Part model, mm, in its own coordinate system. Give positions to 0.01 mm unless a question says otherwise; leave off trailing zeros. One line per question, with ' | ' between items.
```python
from build123d import *

# Parameters (mm, degrees)
SKETCH1_R           = 2.5
BOSS_EXTRUDE1_DEPTH = 240


with BuildPart() as part:
    # Sketch1 → Boss-Extrude1 (new, symmetric)
    with BuildSketch(Plane(origin=(0, 0, 0), x_dir=(1, 0, 0), z_dir=(0, 1, 0))):
        with BuildLine():
            Line((-2.185786438, 3.6), (2.185786438, 3.6))
            Line((2.185786438, 3.6), (5.5, 6.914213562))
            Line((5.5, 6.914213562), (5.5, 8))
            Line((5.5, 8), (3, 8))
            Line((3, 8), (3, 10))
            Line((3, 10), (17, 10))
            Line((17, 10), (17, 8))
            Line((17, 8), (14.5, 8))
            Line((14.5, 8), (14.5, 6.914213562))
            Line((14.5, 6.914213562), (17.814213562, 3.6))
            Line((17.814213562, 3.6), (22.185786438, 3.6))
            Line((22.185786438, 3.6), (25.5, 6.914213562))
            Line((25.5, 6.914213562), (25.5, 8))
            Line((25.5, 8), (23, 8))
            Line((23, 8), (23, 10))
            Line((23, 10), (28.5, 10))
            ThreePointArc((28.5, 10), (29.560660172, 9.560660172), (30, 8.5))
            Line((30, 8.5), (30, 3))
            Line((30, 3), (28, 3))
            Line((28, 3), (28, 5.5))
            Line((28, 5.5), (26.914213562, 5.5))
            Line((26.914213562, 5.5), (23.914213562, 2.5))
            Line((23.914213562, 2.5), (23.914213562, -2.5))
            Line((23.914213562, -2.5), (26.914213562, -5.5))
            Line((26.914213562, -5.5), (28, -5.5))
            Line((28, -5.5), (28, -3))
            Line((28, -3), (30, -3))
            Line((30, -3), (30, -8.5))
            ThreePointArc((30, -8.5), (29.560660172, -9.560660172), (28.5, -10))
            Line((28.5, -10), (23, -10))
            Line((23, -10), (23, -8))
            Line((23, -8), (25.5, -8))
            Line((25.5, -8), (25.5, -6.914213562))
            Line((25.5, -6.914213562), (22.185786438, -3.6))
            Line((22.185786438, -3.6), (17.814213562, -3.6))
            Line((17.814213562, -3.6), (14.5, -6.914213562))
            Line((14.5, -6.914213562), (14.5, -8))
            Line((14.5, -8), (17, -8))
            Line((17, -8), (17, -10))
            Line((17, -10), (3, -10))
            Line((3, -10), (3, -8))
            Line((3, -8), (5.5, -8))
            Line((5.5, -8), (5.5, -6.914213562))
            Line((5.5, -6.914213562), (2.185786438, -3.6))
            Line((2.185786438, -3.6), (-2.185786438, -3.6))
            Line((-2.185786438, -3.6), (-5.5, -6.914213562))
            Line((-5.5, -6.914213562), (-5.5, -8))
            Line((-5.5, -8), (-3, -8))
            Line((-3, -8), (-3, -10))
            Line((-3, -10), (-17, -10))
            Line((-17, -10), (-17, -8))
            Line((-17, -8), (-14.5, -8))
            Line((-14.5, -8), (-14.5, -6.914213562))
            Line((-14.5, -6.914213562), (-17.814213562, -3.6))
            Line((-17.814213562, -3.6), (-22.185786438, -3.6))
            Line((-22.185786438, -3.6), (-25.5, -6.914213562))
            Line((-25.5, -6.914213562), (-25.5, -8))
            Line((-25.5, -8), (-23, -8))
            Line((-23, -8), (-23, -10))
            Line((-23, -10), (-28.5, -10))
            ThreePointArc((-28.5, -10), (-29.560660172, -9.560660172), (-30, -8.5))
            Line((-30, -8.5), (-30, -3))
            Line((-30, -3), (-28, -3))
            Line((-28, -3), (-28, -5.5))
            Line((-28, -5.5), (-26.914213562, -5.5))
            Line((-26.914213562, -5.5), (-23.914213562, -2.5))
            Line((-23.914213562, -2.5), (-23.914213562, 2.5))
            Line((-23.914213562, 2.5), (-26.914213562, 5.5))
            Line((-26.914213562, 5.5), (-28, 5.5))
            Line((-28, 5.5), (-28, 3))
            Line((-28, 3), (-30, 3))
            Line((-30, 3), (-30, 8.5))
            ThreePointArc((-30, 8.5), (-29.560660172, 9.560660172), (-28.5, 10))
            Line((-28.5, 10), (-23, 10))
            Line((-23, 10), (-23, 8))
            Line((-23, 8), (-25.5, 8))
            Line((-25.5, 8), (-25.5, 6.914213562))
            Line((-25.5, 6.914213562), (-22.185786438, 3.6))
            Line((-22.185786438, 3.6), (-17.814213562, 3.6))
            Line((-17.814213562, 3.6), (-14.5, 6.914213562))
            Line((-14.5, 6.914213562), (-14.5, 8))
            Line((-14.5, 8), (-17, 8))
            Line((-17, 8), (-17, 10))
            Line((-17, 10), (-3, 10))
            Line((-3, 10), (-3, 8))
            Line((-3, 8), (-5.5, 8))
            Line((-5.5, 8), (-5.5, 6.914213562))
            Line((-5.5, 6.914213562), (-2.185786438, 3.6))
        make_face()
        with Locations(Location((0, 0, 0), (0, 0, 270))):
            Circle(SKETCH1_R, mode=Mode.SUBTRACT)
        with Locations(Location((20, 0, 0), (0, 0, 270))):
            Circle(SKETCH1_R, mode=Mode.SUBTRACT)
        with Locations(Location((-20, 0, 0), (0, 0, 270))):
            Circle(SKETCH1_R, mode=Mode.SUBTRACT)
        Polygon((7.5, 8), (12.5, 8), (12.5, 6.085786438), (16.085786438, 2.5), (16.085786438, -2.5), (12.5, -6.085786438), (12.5, -8), (7.5, -8), (7.5, -6.085786438), (3.914213562, -2.5), (3.914213562, 2.5), (7.5, 6.085786438), align=None, mode=Mode.SUBTRACT)
        Polygon((-7.5, -6.085786438), (-3.914213562, -2.5), (-3.914213562, 2.5), (-7.5, 6.085786438), (-7.5, 8), (-12.5, 8), (-12.5, 6.085786438), (-16.085786438, 2.5), (-16.085786438, -2.5), (-12.5, -6.085786438), (-12.5, -8), (-7.5, -8), align=None, mode=Mode.SUBTRACT)
    extrude(amount=BOSS_EXTRUDE1_DEPTH, both=True)


solid = part.part
```
1) Pin check, flat tips, straight feed: P1, Ø1, axis at y = -16.5, z = 9, coming from the -X side; P2, Ø1.5, axis at y = -35, z = 1, coming from the -X side; P3, Ø2, axis at x = -20.5, y = -37.5, coming from the -Z side. Stop position of each tip, or through.
Found:
P1: x = -30 | P2: x = -23.91 | P3: z = -3.6
2) Drill centre lines: line 1 (X direction, y = 4, z = 8.5); line 2 (X direction, y = -48.5, z = 0); line 3 (Z direction, x = -24, y = -182.5). Where is each one in solid material? Low to high.
Found:
line 1: -30 to -23, -17 to -3, 3 to 17, 23 to 30 | line 2: -23.91 to -22.5, -17.5 to -16.09, -3.91 to -2.5, 2.5 to 3.91, 16.09 to 17.5, 22.5 to 23.91 | line 3: -10 to -8, -5.41 to -2.59, 2.59 to 5.41, 8 to 10
3) Saw through at A-A (y = 56). State how many separate pieces and enclosed holes the cut face has, and give its area (3 significant figures).
Found:
separate pieces: 1 | enclosed holes: 5 | area: 464 mm2
